from build123d import *

# Parameters (mm, degrees)
BOSS_EXTRUDE1_DEPTH      = 0.0001
BOSS_EXTRUDE1_DEPTH_BACK = 87
SKETCH4_W                = 60
SKETCH4_H                = 60
BOSS_EXTRUDE2_DEPTH      = 2
SKETCH10_W               = 4.646690451
SKETCH10_H               = 22.0001
BOSS_EXTRUDE6_DEPTH      = 4
SKETCH12_W               = 5
SKETCH12_H               = 22.0001
BOSS_EXTRUDE7_DEPTH      = 33.742899166
BOSS_EXTRUDE8_DEPTH      = 4
SKETCH13_R               = 6.25
CUT_EXTRUDE1_DEPTH       = 10
SKETCH14_R               = 8.5
CUT_EXTRUDE2_DEPTH       = 10


with BuildPart() as part:
    # Sketch1 → Boss-Extrude1 (new, two sides: drawn at the far end of the back side and taken through both)
    with BuildSketch(Plane(origin=(0, 0, 0), x_dir=(1, 0, 0), z_dir=(0, 1, 0)).offset(-BOSS_EXTRUDE1_DEPTH_BACK)):
        Polygon((30, 20), (28.5, 20), (28.5, 23.5), (25.3, 23.5), (25.3, 16.871449583), (12.1, 16.871449583), (12.1, 15.181819085), (10.6, 15.181819085), (10.6, 16.685724792), (8.9, 16.685724792), (8.9, 14.346236409), (7.4, 14.346236409), (7.4, 24), (-24, 24), (-24, -24), (7.4, -24), (7.4, -14.346236409), (8.9, -14.346236409), (8.9, -16.685724792), (10.6, -16.685724792), (10.6, -15.181819085), (12.1, -15.181819085), (12.1, -16.871449583), (25.3, -16.871449583), (25.3, -23.5), (28.5, -23.5), (28.5, -20), (30, -20), (30, -30), (-30, -30), (-30, 30), (30, 30), align=None)
    extrude(amount=BOSS_EXTRUDE1_DEPTH + BOSS_EXTRUDE1_DEPTH_BACK)

    # Sketch4 → Boss-Extrude2 (add)
    with BuildSketch(Plane(origin=(0, 0.0001, 0), x_dir=(1, 0, 0), z_dir=(0, 1, 0))):
        Rectangle(SKETCH4_W, SKETCH4_H)
    extrude(amount=BOSS_EXTRUDE2_DEPTH)

    # Sketch10 → Boss-Extrude6 (add)
    with BuildSketch(Plane(origin=(0, 0, 16.871449583), x_dir=(-1, 0, 0), z_dir=(0, 0, -1))):
        with Locations((-9.776654775, -10.99995)):
            Rectangle(SKETCH10_W, SKETCH10_H)
    extrude(amount=BOSS_EXTRUDE6_DEPTH)

    # Sketch12 → Boss-Extrude7 (add)
    with BuildSketch(Plane(origin=(0, 0, 16.871449583), x_dir=(-1, 0, 0), z_dir=(0, 0, -1))):
        with Locations((-22.8, -10.99995)):
            Rectangle(SKETCH12_W, SKETCH12_H)
    extrude(amount=BOSS_EXTRUDE7_DEPTH)

    # Sketch6 → Boss-Extrude8 (add)
    with BuildSketch(Plane.XZ.offset(87)):
        Polygon((28.2, -28), (-28, -28), (-28, 28), (28.2, 28), (28.2, 26), (-26, 26), (-26, -26), (28.2, -26), align=None)
    extrude(amount=BOSS_EXTRUDE8_DEPTH)

    # Sketch13 → Cut-Extrude1 (cut)
    with BuildSketch(Plane.ZY.offset(30)):
        with Locations((14, -7.9999)):
            Circle(SKETCH13_R)
    extrude(amount=-CUT_EXTRUDE1_DEPTH, mode=Mode.SUBTRACT)

    # Sketch14 → Cut-Extrude2 (cut)
    with BuildSketch(Plane(origin=(0, 0, -30), x_dir=(-1, 0, 0), z_dir=(0, 0, -1))):
        with Locations((15, -12.9999)):
            Circle(SKETCH14_R)
        with Locations((15, -36.9999)):
            Circle(SKETCH14_R)
    extrude(amount=-CUT_EXTRUDE2_DEPTH, mode=Mode.SUBTRACT)


solid = part.part
Here's how the part is built. I have some questions about the finished solid (model axes, mm). A direction names the side the tool comes from. Coordinates: 2 decimals unless noted, no trailing zeros. Order: outer loops, then holes, each group sorted by start corner. A loop starts at its lowest first (then second) coordinate and runs counter-clockwise, first axis right, second up.
Item 1: If we section it at D-D on z = -2.5: List the corners of the cut face in (x, y) for me.
Result sheet:
outline: (-30, -87) - (-28, -87) - (-28, -91) - (-26, -91) - (-26, -87) - (-24, -87) - (-24, 0) - (20.3, 0) - (20.3, -22) - (25.3, -22) - (25.3, 0) - (30, 0) - (30, 2) - (-30, 2) - close
Item 2: If we mould it in two halves opening along X, with no side actions, what happens to faces 5 (the face through (-28, -89, 0)), 6 (the face through (0, -43, -30)), 7 (the face through (12.1, -34, 16))? For each: +X half, -X half, draft (parallel to the pull), parting line (faces both ways), or undercut.
Result sheet:
face 5: -X half
face 6: draft
face 7: undercut
Item 3: I need wall thicknesses on line 1 (Y direction, x = -15, z = -25); line 2 (Y direction, x = -15, z = -26.8); line 3 (X direction, y = -45.5, z = 22.5). Which ranges of each line are inside material? Lowest first, please.
Result sheet:
line 1: y = -87 to -45.5, -28.5 to -21.5, -4.5 to 2
line 2: y = -91 to -45.5, -28.5 to -21.5, -4.5 to 2
line 3: x = -30 to -24, 7.4 to 25.3, 28.5 to 30
Item 4: If we section it at A-A on x = -15: List the corners of the cut face in (y, z) for me, plus the area to 3 significant figures.
Result sheet:
outline: (-91, -28) - (-87, -28) - (-87, -30) - (-45.5, -30) - (-45.5, -24) - (-87, -24) - (-87, -26) - (-91, -26) - close; (-91, 26) - (-87, 26) - (-87, 24) - (0, 24) - (0, -24) - (-4.5, -24) - (-4.5, -30) - (2, -30) - (2, 30) - (-87, 30) - (-87, 28) - (-91, 28) - close; (-28.5, -30) - (-21.5, -30) - (-21.5, -24) - (-28.5, -24) - close
area: 976 mm2
Item 5: If we section it at B-B on x = 0: List the corners of the cut face in (y, z) for me.
Result sheet:
outline: (-91, -28) - (-87, -28) - (-87, -30) - (2, -30) - (2, 30) - (-87, 30) - (-87, 28) - (-91, 28) - (-91, 26) - (-87, 26) - (-87, 24) - (0, 24) - (0, -24) - (-87, -24) - (-87, -26) - (-91, -26) - close
Item 6: For faces 1 (the face through (28.2, -89, -27)), 2 (the face through (28.5, -44, -22)), 3 (the face through (0, -89, 28)), 4 (the face through (1, -89, 26)), which set-ups out of +Z, -Z, +X, -X, +Y, -Y let a thin tool reach every point of the face, with its end or its side?
Result sheet:
face 1: +Z, -Z, +X, -Y
face 2: -Y
face 3: +Z, +X, -X, -Y
face 4: +X, -Y
Item 7: For P1, Ø6, axis at x = -11.5, z = -4, coming from the -Y side; P2, Ø24, axis at y = -62.5, z = -2.5, coming from the +X side; P3, Ø1, axis at y = -89.5, z = 26.5, coming from the +X side, each with a flat end and sliding along its axis, tell me the tip position at first contact or that it passes through.
Result sheet:
P1: stops at y = 0
P2: stops at x = 8.9
P3: stops at x = 28.2
